The listing builds one solid part. Answer for the finished solid, in the listing's coordinates (mm). Give positions to 0.01 mm unless a question says otherwise; leave off trailing zeros. Loops run counter-clockwise (first coordinate to the right, second up) from the corner with the lowest first, then second, coordinate; pieces in that order, holes last. Notation, with made-up numbers: (70.5, 67.25) - (124.5, 67.25) arc R31 ccw to (124.5, 93.25) - close; hole circle Ø7 at (-36, 9.5). An arc over 180 degrees is marked (long way). One line per item, written item: value. Start each with the question number.
from build123d import *

# Parameters (mm, degrees)
BOSS_EXTRUDE1_DEPTH         = 6.35
F_3_8_16_TAPPED_HOLE1_D     = 7.9375
F_3_8_16_TAPPED_HOLE1_DEPTH = 6.35
F_3_8_16_TAPPED_HOLE1_TIP   = 2.384665582


with BuildPart() as part:
    # Sketch2 → Boss-Extrude1 (new body)
    with BuildSketch(Plane(origin=(0, 0, 0), x_dir=(1, 0, 0), z_dir=(0, 1, 0))):
        with BuildLine():
            Line((-10.638933845, -0.317978242), (0.0062465, -15.135448057))
            ThreePointArc((0.0062465, -15.135448057), (8.868318086, -16.587580012), (10.320450041, -7.725508427))
            Line((10.320450041, -7.725508427), (0.436752504, 6.032021758))
            Line((0.436752504, 6.032021758), (-10.638933845, 6.032021758))
            Line((-10.638933845, 6.032021758), (-61.438933845, 6.032021758))
            Line((-61.438933845, 6.032021758), (-61.438933845, -0.317978242))
            Line((-61.438933845, -0.317978242), (-10.638933845, -0.317978242))
        make_face()
    extrude(amount=BOSS_EXTRUDE1_DEPTH)

    # 3/8-16 Tapped Hole1
    with Locations(Plane(origin=(0, 6.35, 0), x_dir=(1, 0, 0), z_dir=(0, 1, 0))):
        with Locations((5.218739795, -11.507580012)):
            Hole(F_3_8_16_TAPPED_HOLE1_D / 2, depth=F_3_8_16_TAPPED_HOLE1_DEPTH)
            with Locations((0, 0, -(F_3_8_16_TAPPED_HOLE1_DEPTH + F_3_8_16_TAPPED_HOLE1_TIP / 2))):  # 118° drill point
                Cone(0, F_3_8_16_TAPPED_HOLE1_D / 2, F_3_8_16_TAPPED_HOLE1_TIP, mode=Mode.SUBTRACT)


solid = part.part
1. A cutting plane is placed at B-B (y = 4.75). Determine the outline of the cut face in (x, z).
2. A cutting plane is placed at D-D (z = 1.5). Determine the outline of the cut face in (x, y), plus the area to 3 significant figures.
3. Find the intervals of material crossed by L1, parallel to Z at x = -16, y = 5.75; L2, parallel to X at y = 1, z = 14; L3, parallel to X at y = 2.75, z = 10.75, in increasing order. Write a range as [from, to].
4. Determine the mould class of faces 1 (the flat face through (5.448, 3.131, 0.943)), 2 (the flat face through (-36, 3, 0.318)), 3 (the cylindrical face through (6.08, 3.13, 15.38)), 4 (the flat face through (-20, 0, 0)) for opening direction Z: released by +Z, released by -Z, zero draft, split by the parting line, or undercut.
5. A cutting plane is placed at C-C (x = -40.5). Determine the outline of the cut face in (y, z), plus the area to 3 significant figures.
6. A cutting plane is placed at A-A (z = 12.25). Determine the outline of the cut face in (x, y), plus the area to 3 significant figures.
7. Flat-ended cylindrical pins translate along their axes: pin 1 (3 mm diameter, centred on y = 2, z = -2.5, fed in from +X); pin 2 (1.9 mm diameter, centred on x = -37.5, y = 3, fed in from +Z). Find the tip coordinate at first contact, or state that the pin passes through.
Results below:
1. outline: (-61.44, -6.03) - (0.44, -6.03) - (10.32, 7.73) arc R6.35 ccw to (0.01, 15.14) - (-10.64, 0.32) - (-61.44, 0.32) - close; hole circle Ø7.94 at (5.22, 11.51)
2. outline: (-9.79, 0) - (5.85, 0) - (5.85, 6.35) - (-9.79, 6.35) - close
2. area: 99.3 mm^2
3. L1: z = [-6.03, 0.32]
3. L2: x = [-0.81, 2.13], [8.31, 10.97]
3. L3: x = [-3.14, 1.32], [9.11, 11.48]
4. face 1: released by -Z
4. face 2: released by +Z
4. face 3: undercut
4. face 4: zero draft
5. outline: (0, -6.03) - (6.35, -6.03) - (6.35, 0.32) - (0, 0.32) - close
5. area: 40.3 mm^2
6. outline: (-2.07, 0) - (1.32, 0) - (1.32, 6.35) - (-2.07, 6.35) - close; (9.12, 0) - (11.46, 0) - (11.46, 6.35) - (9.12, 6.35) - close
6. area: 36.4 mm^2
7. pin 1: stops at x = 4.05
7. pin 2: stops at z = 0.32
